```python
from build123d import *

# Parameters (mm, degrees)
BOSS_EXTRUDE1_DEPTH = 15.24
SKETCH2_R           = 20
BOSS_EXTRUDE2_DEPTH = 3
BOSS_EXTRUDE3_START = 18.24
BOSS_EXTRUDE3_DEPTH = 15.24
FILLET1_R           = 2
SKETCH3_W           = 35.8896148
SKETCH3_H           = 21.37412809
CUT_EXTRUDE1_DEPTH  = 51.878317112
CHAMFER2_SIZE       = 1.5
SKETCH5_W           = 51.439810339
SKETCH5_H           = 15.927026311
CUT_EXTRUDE3_DEPTH  = 50.49162642


with BuildPart() as part:
    # Sketch1 → Boss-Extrude1 (new body)
    with BuildSketch(Plane(origin=(0, 0, 0), x_dir=(1, 0, 0), z_dir=(0, 1, 0))):
        Polygon((5.9375, 10.28405167), (-5.9375, 10.28405167), (-11.875, 0), (-5.9375, -10.28405167), (5.9375, -10.28405167), (11.875, 0), align=None)
    extrude(amount=BOSS_EXTRUDE1_DEPTH)

    # Sketch2 → Boss-Extrude2 (add)
    with BuildSketch(Plane(origin=(0, 15.24, 0), x_dir=(1, 0, 0), z_dir=(0, 1, 0))):
        with Locations(Location((0, 0, 0), (0, 0, 270))):
            Circle(SKETCH2_R)
    extrude(amount=BOSS_EXTRUDE2_DEPTH)

    # Sketch1<2> → Boss-Extrude3 (add)
    with BuildSketch(Plane(origin=(0, 0, 0), x_dir=(1, 0, 0), z_dir=(0, 1, 0)).offset(BOSS_EXTRUDE3_START)):
        Polygon((5.9375, 10.28405167), (-5.9375, 10.28405167), (-11.875, 0), (-5.9375, -10.28405167), (5.9375, -10.28405167), (11.875, 0), align=None)
    extrude(amount=BOSS_EXTRUDE3_DEPTH)

    # Fillet1
    fillet1_edges = [part.edges().sort_by_distance(p)[0] for p in [
        (11.875, 7.62, 0),
        (5.9375, 7.62, 10.28405167),
        (-5.9375, 7.62, 10.28405167),
        (-11.875, 7.62, 0),
        (-5.9375, 7.62, -10.28405167),
        (5.9375, 7.62, -10.28405167),
        (-5.9375, 25.86, 10.28405167),
        (5.9375, 25.86, 10.28405167),
        (11.875, 25.86, 0),
        (5.9375, 25.86, -10.28405167),
        (-5.9375, 25.86, -10.28405167),
        (-11.875, 25.86, 0),
    ]]
    fillet(fillet1_edges, radius=FILLET1_R)

    # Sketch3 → Cut-Extrude1 (cut, through all)
    with BuildSketch(Plane(origin=(-8.90625, 0, -5.142025835), x_dir=(-0.5000000000000004, 0, 0.8660254037844385), z_dir=(-0.8660254037844384, 0, -0.5000000000000003))):
        with Locations((0.576480633, 22.756432149)):
            Rectangle(SKETCH3_W, SKETCH3_H)
    extrude(amount=CUT_EXTRUDE1_DEPTH, mode=Mode.SUBTRACT)

    # Chamfer2
    chamfer2_edges = [part.edges().sort_by_distance(p)[0] for p in [
        (0, 0, -10.28405167),
        (8.90625, 0, -5.142025835),
        (8.90625, 0, 5.142025835),
        (0, 0, 10.28405167),
        (-8.90625, 0, 5.142025835),
        (-8.90625, 0, -5.142025835),
        (11.565598923, 0, 0),
        (5.782799462, 0, 10.016102478),
        (-5.782799462, 0, 10.016102478),
        (-11.565598923, 0, 0),
        (-5.782799462, 0, -10.016102478),
        (5.782799462, 0, -10.016102478),
        (0, 33.48, -10.28405167),
        (8.90625, 33.48, -5.142025835),
        (0, 33.48, 10.28405167),
        (8.90625, 33.48, 5.142025835),
        (-8.90625, 33.48, -5.142025835),
        (-8.90625, 33.48, 5.142025835),
        (11.565598923, 33.48, 0),
        (5.782799462, 33.48, 10.016102478),
        (-5.782799462, 33.48, 10.016102478),
        (-11.565598923, 33.48, 0),
        (-5.782799462, 33.48, -10.016102478),
        (5.782799462, 33.48, -10.016102478),
    ]]
    chamfer(chamfer2_edges, length=CHAMFER2_SIZE)

    # Sketch5 → Cut-Extrude3 (cut, through all)
    with BuildSketch(Plane(origin=(8.90625, 0, 5.142025835), x_dir=(0.5000000000000004, 0, -0.8660254037844384), z_dir=(0.8660254037844384, 0, 0.5000000000000004))):
        with Locations((-1.041050082, 20.809011755)):
            Rectangle(SKETCH5_W, SKETCH5_H)
    extrude(amount=CUT_EXTRUDE3_DEPTH, mode=Mode.SUBTRACT)


solid = part.part
```
The model under review builds one solid part; all positions refer to its coordinate system, in mm. A direction names the side the tool comes from. Round coordinates to 2 decimals unless told otherwise and drop trailing zeros. Loops run counter-clockwise (first coordinate to the right, second up) from the corner with the lowest first, then second, coordinate; pieces in that order, holes last. Notation, with made-up numbers: (88, 67) -> (117, 67) arc R34 cw to (117, 99) -> close; hole circle Ø2 at (34, -13). An arc over 180 degrees is marked (long way). Answer in a Markdown table with one row per item.
1) For pin 1 Ø1 at (y, z) = (26.5, 7.5) entering from -X; pin 2 Ø4 at (y, z) = (17, 5) entering from -X; pin 3 Ø5 at (y, z) = (22, -2) entering from +X; pin 4 Ø10.5 at (x, y) = (0.5, 23) entering from -Z, all flat-tipped, find the tip position at first contact; note any pin that passes through.
Taken from the geometry:
| item | result |
|---|---|
| pin 1 | stops at x = -7.83 |
| pin 2 | stops at x = -15.92 |
| pin 3 | stops at x = 11.57 |
| pin 4 | stops at z = -20 |
2) Consider section C-C, the plane x = 4. Write out the cut boundary in (y, z), plus the area to 3 significant figures.
Taken from the geometry:
| item | result |
|---|---|
| outline | (0, -8.78) -> (1.5, -10.28) -> (15.24, -10.28) -> (15.24, -19.6) -> (18.24, -19.6) -> (18.24, -10.28) -> (31.98, -10.28) -> (33.48, -8.78) -> (33.48, 8.78) -> (31.98, 10.28) -> (18.24, 10.28) -> (18.24, 13.64) -> (15.24, 13.64) -> (15.24, 10.28) -> (1.5, 10.28) -> (0, 8.78) -> close |
| area | 722 mm² |
3) Wall thickness on line 1 along Y through (x, z) = (0, -15); line 2 along Z through (x, y) = (3, 31.5); line 3 along Y through (x, z) = (0, 9): over which ranges is each line inside the solid? List them lowest first.
Taken from the geometry:
| item | result |
|---|---|
| line 1 | y = 15.24 to 18.24 |
| line 2 | z = -10.28 to 10.28 |
| line 3 | y = 0.22 to 33.26 |
4) Consider section A-A, the plane y = 3.5. Write out the cut boundary in (x, z), plus the area to 3 significant figures.
Taken from the geometry:
| item | result |
|---|---|
| outline | (-11.3, -1) -> (-6.51, -9.28) arc R2 ccw to (-4.78, -10.28) -> (4.78, -10.28) arc R2 ccw to (6.51, -9.28) -> (11.3, -1) arc R2 ccw to (11.3, 1) -> (6.51, 9.28) arc R2 ccw to (4.78, 10.28) -> (-4.78, 10.28) arc R2 ccw to (-6.51, 9.28) -> (-11.3, 1) arc R2 ccw to start |
| area | 365 mm² |
5) Consider section D-D, the plane y = 17. Write out the cut boundary in (x, z).
Taken from the geometry:
| item | result |
|---|---|
| outline | (-17.48, 9.71) -> (-0.33, -20) arc R20 ccw to (17.48, -9.71) -> (0.33, 20) arc R20 ccw to start |
6) Consider section B-B, the plane z = -5. Write out the cut boundary in (x, y), plus the area to 3 significant figures.
Taken from the geometry:
| item | result |
|---|---|
| outline | (-8.99, 1.5) -> (-7.26, 0) -> (7.26, 0) -> (8.99, 1.5) -> (8.99, 15.24) -> (14.76, 15.24) -> (14.76, 18.24) -> (8.99, 18.24) -> (8.99, 31.98) -> (7.26, 33.48) -> (-7.26, 33.48) -> (-8.99, 31.98) -> close |
| area | 614 mm² |
7) Tool access review of faces 1 (the flat face through (0, 25, 10.284)), 2 (the cylindrical face through (5.77, 25.206, 10.023)), 3 (the flat face through (-8.94, 25.01, 5.08)): name each direction out of +Z, -Z, +X, -X, +Y, -Y from which nothing blocks a thin tool from reaching the whole face with its end or side.
Taken from the geometry:
| item | result |
|---|---|
| face 1 | +Z, +X, -X, +Y |
| face 2 | +Z, +X, +Y |
| face 3 | +Z, -X, +Y |
